Build history of the part. All positions in model axes, mm. Face numbers are marked on the shaded views. A direction names the side the tool comes from. Round coordinates to 2 decimals unless told otherwise and drop trailing zeros. Loops run counter-clockwise (first coordinate to the right, second up) from the corner with the lowest first, then second, coordinate; pieces in that order, holes last. Notation, with made-up numbers: M 8.5,52 L 60.5,52 A15 ccw 60.5,81 Z; hole C 25.5,-12.5 d2. An arc over 180 degrees is marked long. Use one line per item in the form item = value. Start each with the question number.
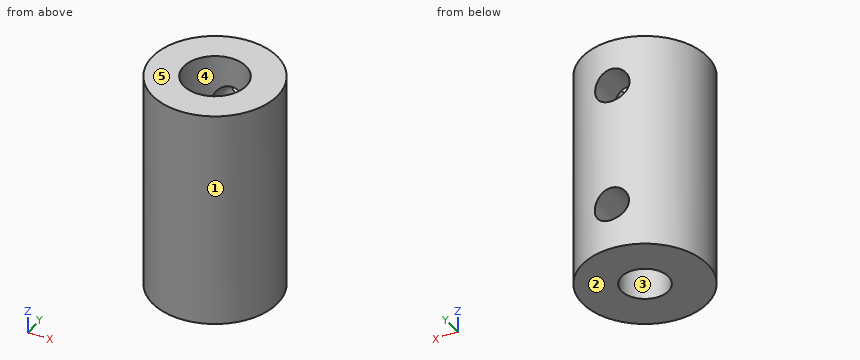
```python
from build123d import *

# Parameters (mm, degrees)
SKETCH1_R                           = 6.35
BOSS_EXTRUDE1_DEPTH                 = 22.225
SKETCH2_R                           = 3.175
THICK_DEPTH                         = 12.7
SKETCH3_R                           = 2.38125
THIN_DEPTH                          = 12.7
F_8_32_TAPPED_HOLE2_REACH           = 24.512
F_8_32_TAPPED_HOLE2_BORE_R          = 1.7272
F_8_32_TAPPED_HOLE2_ON_FACE_2_REACH = 24.515
F_8_32_TAPPED_HOLE2_BORE_2_R        = 1.7272


with BuildPart() as part:
    # Sketch1 → Boss-Extrude1 (new body)
    with BuildSketch(Plane.XY):
        Circle(SKETCH1_R)
    extrude(amount=BOSS_EXTRUDE1_DEPTH)

    # Sketch2 → Thick (cut)
    with BuildSketch(Plane.XY.offset(22.225)):
        Circle(SKETCH2_R)
    extrude(amount=-THICK_DEPTH, mode=Mode.SUBTRACT)

    # Sketch3 → Thin (cut)
    with BuildSketch(Plane(origin=(0, 0, 0), x_dir=(-1, 0, 0), z_dir=(0, 0, -1))):
        Circle(SKETCH3_R)
    extrude(amount=-THIN_DEPTH, mode=Mode.SUBTRACT)

    # #8-32 Tapped Hole2 bore (on position points) → #8-32 Tapped Hole2 (cut, up to next)
    with BuildSketch(Plane(origin=(-0.017626293, 6.349975536, 17.4625), x_dir=(0.999996147476, 0.002775794184, 0), z_dir=(-0.002775794184, 0.999996147476, 0)), mode=Mode.PRIVATE) as f_8_32_tapped_hole2_sk1:
        Circle(F_8_32_TAPPED_HOLE2_BORE_R)
    f_8_32_tapped_hole2_tool1 = extrude(f_8_32_tapped_hole2_sk1.sketch, amount=-F_8_32_TAPPED_HOLE2_REACH, mode=Mode.PRIVATE) & part.part
    add(f_8_32_tapped_hole2_tool1.solids().sort_by_distance((-0.017626, 6.349976, 17.4625))[0], mode=Mode.SUBTRACT)

    # #8-32 Tapped Hole2 bore 2 (on position points) → #8-32 Tapped Hole2 on face 2 (cut, up to next)
    with BuildSketch(Plane(origin=(0.028231467, 6.349937243, 4.7625), x_dir=(0.999990116491, -0.004446000518, 0), z_dir=(0.004446000518, 0.999990116491, 0)), mode=Mode.PRIVATE) as f_8_32_tapped_hole2_on_face_2_sk1:
        Circle(F_8_32_TAPPED_HOLE2_BORE_2_R)
    f_8_32_tapped_hole2_on_face_2_tool1 = extrude(f_8_32_tapped_hole2_on_face_2_sk1.sketch, amount=-F_8_32_TAPPED_HOLE2_ON_FACE_2_REACH, mode=Mode.PRIVATE) & part.part
    add(f_8_32_tapped_hole2_on_face_2_tool1.solids().sort_by_distance((0.028231, 6.349937, 4.7625))[0], mode=Mode.SUBTRACT)


solid = part.part
```
Q1. Tool access for the marked faces 4 and 5: list every direction of +Z, -Z, +X, -X, +Y, -Y with a clear straight run to the whole face (end or side of a thin tool).
Q2. Saw through at D-D (y = -1.75). Give the cut face in (x, z) (3 decimals), and give its area (3 significant figures).
Q3. Saw through at A-A (y = 0). Give the cut face in (x, z) (3 decimals).
Q4. Saw through at B-B (z = 20.5). Give the cut face in (x, y) (3 decimals), and give its area (3 significant figures).
Q5. Drop flat-ended pins along their axis: P1, Ø5, axis at x = 0.5, y = 1, coming from the +Z side (3 decimals); P2, Ø1, axis at y = -3.5, z = 5, coming from the +X side; P3, Ø1, axis at y = 1, z = 16.5, coming from the -X side; P4, Ø4, axis at x = 0, y = 0, coming from the -Z side. Give the stop position or say it passes through.
Q6. Saw through at C-C (x = 0). Give the number of separate pieces and of enclosed holes in the cut face, and give its area (3 significant figures).
Q7. Wall check: probe 1 along Y at (x, z) = (0, 13) (3 decimals); probe 2 along Z at (x, y) = (-0.75, 4.25) (3 decimals); probe 3 along Y at (x, z) = (0, 7.5). Give the ranges that are in metal, low to high.
Q8. Pull direction Y, two halves, no side cores. Call the marked faces 1, 2 and 3: pulls with the +Y half, pulls with the -Y half, needs draft (parallel to the pull), parting line crosses it, or undercut.
Filled in:
q1.face_4 = +Z
q1.face_5 = +Z, +X, -X, +Y, -Y
q2.outline = M -6.104,0 L -1.615,0 L -1.615,9.525 L -2.649,9.525 L -2.649,22.225 L -6.104,22.225 Z; M 1.615,0 L 6.104,0 L 6.104,22.225 L 2.649,22.225 L 2.649,9.525 L 1.615,9.525 Z
q2.area = 173 mm²
q3.outline = M -6.35,0 L -2.381,0 L -2.381,9.525 L -3.175,9.525 L -3.175,22.225 L -6.35,22.225 Z; M 2.381,0 L 6.35,0 L 6.35,22.225 L 3.175,22.225 L 3.175,9.525 L 2.381,9.525 Z
q4.outline = C 0,0 d12.7; hole C 0,0 d6.35
q4.area = 95.0 mm²
q5.P1 = 22.225
q5.P2 = 5.6
q5.P3 = -6.33
q5.P4 = through
q6.separate_pieces = 4
q6.enclosed_holes = 0
q6.area = 132 mm²
q7.probe_1 = -6.35 to -3.175, 3.175 to 6.35
q7.probe_2 = 0 to 3.216, 6.309 to 15.901, 19.024 to 22.225
q7.probe_3 = -6.35 to -2.38, 2.38 to 6.35
q8.face_1 = parting line crosses it
q8.face_2 = needs draft
q8.face_3 = undercut
